```python
from build123d import *

# Parameters (mm, degrees)
SKETCH1_W               = 30
SKETCH1_H               = 75
MAIN_BLOCK_DEPTH        = 25
FRAME_HOLE_REACH        = 82.467
SKETCH2_R               = 5
EM_ROD_HOLES_REACH      = 56.141
EM_ROD_HOLES_SKETCH_R   = 5
BOSS_EXTRUDE1_DEPTH     = 10
CUT_EXTRUDE1_DEPTH      = 52.53882032
CUT_EXTRUDE1_DEPTH_BACK = 52.53882032
SKETCH5_W               = 30
SKETCH5_H               = 75


with BuildPart() as part:
    # Sketch1 → Main Block (new, symmetric)
    with BuildSketch(Plane(origin=(0, 0, 0), x_dir=(1, 0, 0), z_dir=(0, 1, 0))):
        Rectangle(SKETCH1_W, SKETCH1_H)
    extrude(amount=MAIN_BLOCK_DEPTH, both=True)

    # Sketch2 → Frame Hole (cut, up to next)
    with BuildSketch(Plane.XY.offset(37.5), mode=Mode.PRIVATE) as frame_hole_sk1:
        with Locations((0, -15)):
            Circle(SKETCH2_R)
    frame_hole_tool1 = extrude(frame_hole_sk1.sketch, amount=-FRAME_HOLE_REACH, mode=Mode.PRIVATE) & part.part
    add(frame_hole_tool1.solids().sort_by_distance((0, -15, 37.5))[0], mode=Mode.SUBTRACT)

    # EM Rod Holes Sketch → EM Rod Holes (cut, up to next)
    with BuildSketch(Plane(origin=(15, 0, 0), x_dir=(0, 0, -1), z_dir=(1, 0, 0)), mode=Mode.PRIVATE) as em_rod_holes_sk1:
        with Locations((-15, 15)):
            Circle(EM_ROD_HOLES_SKETCH_R)
    em_rod_holes_tool1 = extrude(em_rod_holes_sk1.sketch, amount=-EM_ROD_HOLES_REACH, mode=Mode.PRIVATE) & part.part
    # EM Rod Holes Sketch → EM Rod Holes (cut, up to next)
    with BuildSketch(Plane(origin=(15, 0, 0), x_dir=(0, 0, -1), z_dir=(1, 0, 0)), mode=Mode.PRIVATE) as em_rod_holes_sk2:
        with Locations((15, 15)):
            Circle(EM_ROD_HOLES_SKETCH_R)
    em_rod_holes_tool2 = extrude(em_rod_holes_sk2.sketch, amount=-EM_ROD_HOLES_REACH, mode=Mode.PRIVATE) & part.part
    add(em_rod_holes_tool1.solids().sort_by_distance((15, 15, 15))[0], mode=Mode.SUBTRACT)
    add(em_rod_holes_tool2.solids().sort_by_distance((15, 15, -15))[0], mode=Mode.SUBTRACT)

    # Sketch4 → Boss-Extrude1 (add)
    with BuildSketch(Plane.XZ.offset(25)):
        Polygon((-15, 33.3), (-15, 37.5), (-25, 37.5), (-25, 36.4), (-24, 36.4), (-18, 36.4), (-18, 34.4), (-24, 34.4), (-25, 34.4), (-25, 33.3), align=None)
        with BuildLine():
            Line((-24, 36.4), (-25, 36.4))
            ThreePointArc((-25, 36.4), (-24.612310563, 36.25075775), (-24.2, 36.2))
            ThreePointArc((-24.2, 36.2), (-24.058578644, 36.258578644), (-24, 36.4))
        make_face()
        with BuildLine():
            ThreePointArc((-24.2, 34.6), (-24.612310563, 34.54924225), (-25, 34.4))
            Line((-25, 34.4), (-24, 34.4))
            ThreePointArc((-24, 34.4), (-24.058578644, 34.541421356), (-24.2, 34.6))
        make_face()
    extrude(amount=-BOSS_EXTRUDE1_DEPTH)

    # Sketch5 → Cut-Extrude1 (cut, two sides: drawn at the far end of the back side and taken through both)
    with BuildSketch(Plane(origin=(0, 0, 0), x_dir=(1, 0, 0), z_dir=(0, 1, 0)).offset(-CUT_EXTRUDE1_DEPTH_BACK)):
        Rectangle(SKETCH5_W, SKETCH5_H)
    extrude(amount=CUT_EXTRUDE1_DEPTH + CUT_EXTRUDE1_DEPTH_BACK, mode=Mode.SUBTRACT)


solid = part.part
```
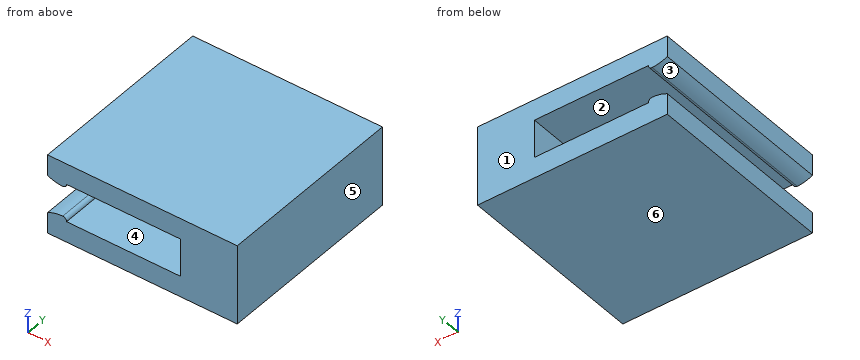
Check sheet for the modelled part. Datum: model origin and axes. Units: mm. Face numbers are marked on the shaded views. A direction names the side the tool comes from. Coordinates: 2 decimals unless noted, no trailing zeros. Loops run counter-clockwise (first coordinate to the right, second up) from the corner with the lowest first, then second, coordinate; pieces in that order, holes last.
1) Sectioned sample at B-B (y = -17). Record the boundary of the cut face in (x, z).
2) Release check for a two-part mould opening along X. For the marked faces 4, 5 and 6 record: released by +X, released by -X, zero draft, split by the parting line, or undercut.
3) Sectioned sample at C-C (z = 34.9). Record the boundary of the cut face in (x, y), and give its area (3 significant figures).
4) Material ranges on probe 1 along Z at (x, y) = (-22.75, -22.5); probe 2 along X at (y, z) = (-18.5, 35.9), recorded low to high.
5) Sectioned sample at A-A (x = -18.25). Record the boundary of the cut face in (y, z).
6) Gauge pin test, flat end, axial feed: pin 1 (0.6 mm diameter, centred on y = -19.5, z = 35.5, fed in from -X). Record the tip position at first contact, or that the pin passes through.
7) Access from +Z, -Z, +X, -X, +Y, -Y to the whole of each face (thin tool, end or side, straight path). Record for the marked faces 1, 2 and 3.
Check sheet entries:
1. outline: (-25, 33.3) - (-15, 33.3) - (-15, 37.5) - (-25, 37.5) - (-25, 36.4) arc R1.7 ccw to (-24.2, 36.2) arc R0.2 ccw to (-24, 36.4) - (-18, 36.4) - (-18, 34.4) - (-24, 34.4) arc R0.2 ccw to (-24.2, 34.6) arc R1.7 ccw to (-25, 34.4) - close
2. face 4: undercut
2. face 5: released by +X
2. face 6: zero draft
3. outline: (-18, -25) - (-15, -25) - (-15, -15) - (-18, -15) - close
3. area: 30.0 mm2
4. probe 1: z = 33.3 to 34.4, 36.4 to 37.5
4. probe 2: x = -18 to -15
5. outline: (-25, 33.3) - (-15, 33.3) - (-15, 34.4) - (-25, 34.4) - close; (-25, 36.4) - (-15, 36.4) - (-15, 37.5) - (-25, 37.5) - close
6. pin 1: stops at x = -18
7. face 1: +Z, -Z, +X, -X, +Y
7. face 2: +Y, -Y
7. face 3: -X, +Y, -Y
